Part model, mm, in its own coordinate system. Give positions to 0.01 mm unless a question says otherwise; leave off trailing zeros. Write each loop counter-clockwise with the first axis right and the second up, starting at its lowest first coordinate (ties: lowest second). Pieces come first, ordered by that corner, then holes. Notation, with made-up numbers: M 2.25,40 L 46.25,40 A22 cw 46.25,53 Z; hole C -27,88.25 d10. An arc over 180 degrees is marked long. Use a Markdown table: item, result.
```python
from build123d import *

# Parameters (mm, degrees)
SKETCH1_W           = 108
SKETCH1_H           = 360
SKETCH1_R           = 13
SKETCH1_R_2         = 1.5
SKETCH1_R_3         = 2
BOSS_EXTRUDE1_DEPTH = 8
FILLET1_R           = 12


with BuildPart() as part:
    # Sketch1 → Boss-Extrude1 (new body)
    with BuildSketch(Plane(origin=(0, 0, 0), x_dir=(1, 0, 0), z_dir=(0, 1, 0))):
        with Locations((-1, 0)):
            Rectangle(SKETCH1_W, SKETCH1_H)
        with Locations(Location((0, 125, 0), (0, 0, 270))):
            Circle(SKETCH1_R, mode=Mode.SUBTRACT)
        with Locations(Location((-42, 83, 0), (0, 0, 270))):
            Circle(SKETCH1_R_2, mode=Mode.SUBTRACT)
        with Locations(Location((-42, 167, 0), (0, 0, 270))):
            Circle(SKETCH1_R_2, mode=Mode.SUBTRACT)
        with Locations(Location((42, 167, 0), (0, 0, 270))):
            Circle(SKETCH1_R_2, mode=Mode.SUBTRACT)
        with Locations(Location((42, 83, 0), (0, 0, 270))):
            Circle(SKETCH1_R_2, mode=Mode.SUBTRACT)
        with Locations(Location((-12.904698757, 112.095301243, 0), (0, 0, 270))):
            Circle(SKETCH1_R_3, mode=Mode.SUBTRACT)
        with Locations(Location((-12.904698757, 137.904698757, 0), (0, 0, 270))):
            Circle(SKETCH1_R_3, mode=Mode.SUBTRACT)
        with Locations(Location((12.904698757, 137.904698757, 0), (0, 0, 270))):
            Circle(SKETCH1_R_3, mode=Mode.SUBTRACT)
        with Locations(Location((12.904698757, 112.095301243, 0), (0, 0, 270))):
            Circle(SKETCH1_R_3, mode=Mode.SUBTRACT)
        with Locations(Location((-42, 5, 0), (0, 0, 270))):
            Circle(SKETCH1_R_2, mode=Mode.SUBTRACT)
        with Locations(Location((-42, -73, 0), (0, 0, 270))):
            Circle(SKETCH1_R_2, mode=Mode.SUBTRACT)
        with Locations(Location((-42, -151, 0), (0, 0, 270))):
            Circle(SKETCH1_R_2, mode=Mode.SUBTRACT)
        with Locations(Location((42, -151, 0), (0, 0, 90))):
            Circle(SKETCH1_R_2, mode=Mode.SUBTRACT)
        with Locations(Location((42, -73, 0), (0, 0, 90))):
            Circle(SKETCH1_R_2, mode=Mode.SUBTRACT)
        with Locations(Location((42, 5, 0), (0, 0, 90))):
            Circle(SKETCH1_R_2, mode=Mode.SUBTRACT)
    extrude(amount=BOSS_EXTRUDE1_DEPTH)

    # Fillet1
    fillet1_edges = [part.edges().sort_by_distance(p)[0] for p in [
        (53, 4, 180),
        (-55, 4, 180),
        (-55, 4, -180),
        (53, 4, -180),
    ]]
    fillet(fillet1_edges, radius=FILLET1_R)


solid = part.part
```
1. Drill centre lines: L1, parallel to X at y = 5.5, z = 73; L2, parallel to Z at x = -4, y = 1. Where is each one in solid material? Low to high.
Findings below:
| item | result |
|---|---|
| L1 | -55 to -43.5, -40.5 to 40.5, 43.5 to 53 |
| L2 | -180 to -137.37, -112.63 to 180 |
2. Two-plate mould, pull along Z, no slides. Class faces 1 (the cylindrical face through (-51.58, 4.06, 176.39)), 2 (the cylindrical face through (3.9, 3.9, -112.6)), 3 (the flat face through (-2, 8, -3)), 4 (the cylindrical face through (49.39, 4.06, -176.58)): released by +Z, released by -Z, zero draft, split by the parting line, or undercut.
Findings below:
| item | result |
|---|---|
| face 1 | released by +Z |
| face 2 | undercut |
| face 3 | zero draft |
| face 4 | released by -Z |
3. Drop flat-ended pins along their axis: P1, Ø4, axis at x = 42, z = 151, coming from the +Y side; P2, Ø2.5, axis at x = 42, z = -83, coming from the +Y side. Give the stop position or say it passes through.
Findings below:
| item | result |
|---|---|
| P1 | y = 8 |
| P2 | through |
4. Cut at C-C, the plane y = 3.5. State how many separate pieces and enclosed holes the cut face has, then the cut area to 3 significant figures.
Findings below:
| item | result |
|---|---|
| separate pieces | 1 |
| enclosed holes | 15 |
| area | 38,100 mm2 |
5. Cut at A-A, the plane z = -125. Give the cut face in (x, y), then the cut area to 3 significant figures.
Findings below:
| item | result |
|---|---|
| outline | M -55,0 L -13,0 L -13,8 L -55,8 Z; M 13,0 L 53,0 L 53,8 L 13,8 Z |
| area | 656 mm2 |
6. Cut at B-B, the plane x = 0. Give the cut face in (y, z).
Findings below:
| item | result |
|---|---|
| outline | M 0,-180 L 8,-180 L 8,-138 L 0,-138 Z; M 0,-112 L 8,-112 L 8,180 L 0,180 Z |
